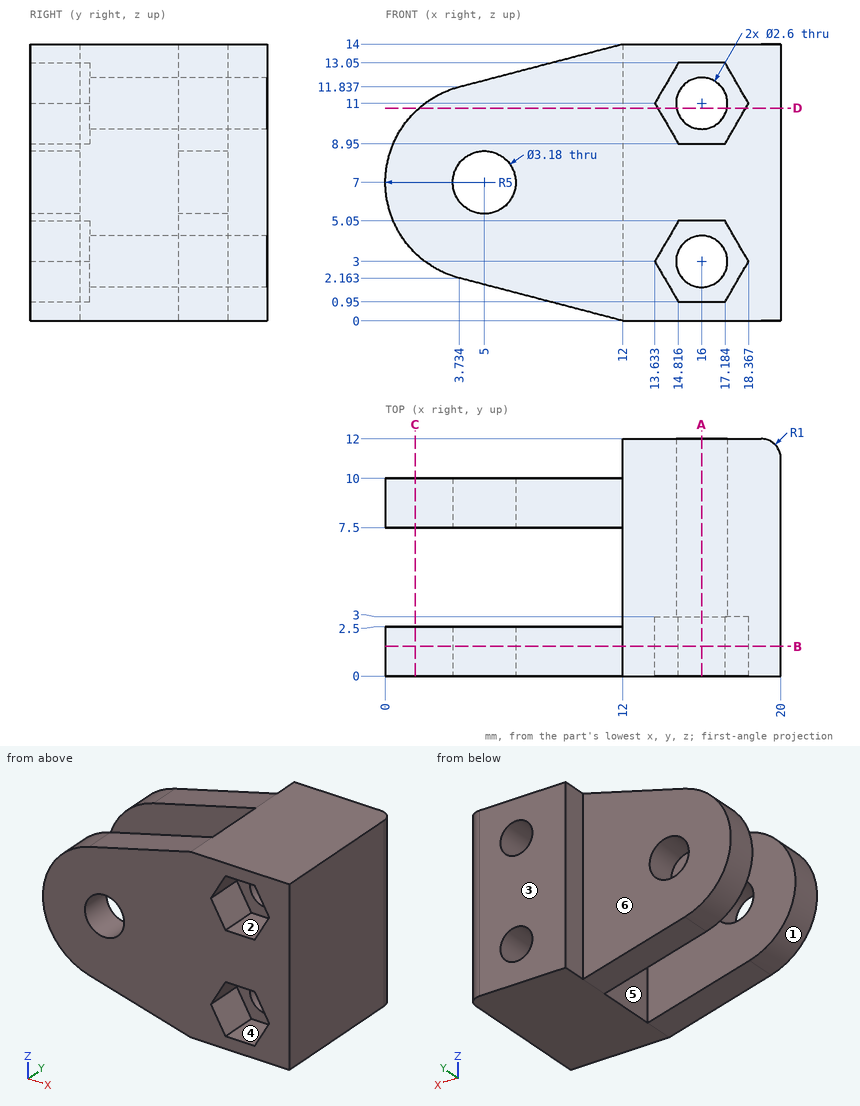
Study the drawing (mm; zero at the part's minimum x, y, z) and answer. A direction names the side the tool comes from. Give positions to 0.01 mm unless a question says otherwise; leave off trailing zeros. Order: outer loops, then holes, each group sorted by start corner. A loop starts at its lowest first (then second) coordinate and runs counter-clockwise, first axis right, second up. Notation, with made-up numbers: (-37.5, 54.25) - (-30.5, 54.25) arc R23 cw to (-30.5, 66.25) - close; hole circle Ø9 at (-29, 83). An arc over 180 degrees is marked (long way). Answer in a Markdown table with one row per item. Add a question column.
Q1. Which of the six approach directions +Z, -Z, +X, -X, +Y, -Y give full straight-line access (tool end or side, diameter ignored) to the marked faces 4, 5 and 6?
Q2. The part is cut by section B-B (y = 1.5). Give the number of separate pieces and of enclosed holes in the cut face.
Q3. The part is cut by section C-C (x = 1.5). Determine the outline of the cut face in (y, z), then the cut area to 3 significant figures.
Q4. Find the intervals of material crossed by line 1 along Z through (x, y) = (16, 9.25); line 2 along Z through (x, y) = (16.25, 1.5); line 3 along Y through (x, z) = (7.75, 6), in increasing order. Write a range as [from, to].
Q5. For a pull along X with two mould halves and no side action, classify the marked faces 1, 2 and 3 as released by +X, released by -X, zero draft, split by the parting line, or undercut.
Q6. The part is cut by section D-D (z = 10.75). Determine the outline of the cut face in (x, y) (1 decimal).
Q7. The part is cut by section A-A (x = 16). Determine the outline of the cut face in (y, z).
Q8. Given P1, Ø5, axis at x = 2, z = 8.5, coming from the +Y side; P2, Ø4, axis at x = 8, y = 7.5, coming from the -Z side; P3, Ø1, axis at y = 11, z = 6, coming from the -X side, each flat-ended and moving along its own axis, determine where each tip first touches the part or whether it passes through.
Determined:
| question | item | result |
|---|---|---|
| 1 | face 4 | -Y |
| 1 | face 5 | +Z, -Z, -X |
| 1 | face 6 | +Z, -Z, -X, +Y |
| 2 | separate pieces | 1 |
| 2 | enclosed holes | 3 |
| 3 | outline | (0, 3.43) - (2.5, 3.43) - (2.5, 10.57) - (0, 10.57) - close; (7.5, 3.43) - (10, 3.43) - (10, 10.57) - (7.5, 10.57) - close |
| 3 | area | 35.7 mm² |
| 4 | line 1 | z = [0, 1.7], [4.3, 9.7], [12.3, 14] |
| 4 | line 2 | z = [0, 0.95], [5.05, 8.95], [13.05, 14] |
| 4 | line 3 | y = [0, 2.5], [7.5, 10] |
| 5 | face 1 | released by -X |
| 5 | face 2 | undercut |
| 5 | face 3 | zero draft |
| 6 | outline | (1.7, 0) - (13.8, 0) - (13.8, 3) - (14.7, 3) - (14.7, 12) - (12, 12) - (12, 10) - (1.7, 10) - (1.7, 7.5) - (12, 7.5) - (12, 2.5) - (1.7, 2.5) - close; (17.3, 3) - (18.2, 3) - (18.2, 0) - (20, 0) - (20, 11) arc R1 ccw to (19, 12) - (17.3, 12) - close |
| 7 | outline | (0, 0) - (12, 0) - (12, 1.7) - (3, 1.7) - (3, 0.95) - (0, 0.95) - close; (0, 5.05) - (3, 5.05) - (3, 4.3) - (12, 4.3) - (12, 9.7) - (3, 9.7) - (3, 8.95) - (0, 8.95) - close; (0, 13.05) - (3, 13.05) - (3, 12.3) - (12, 12.3) - (12, 14) - (0, 14) - close |
| 8 | P1 | stops at y = 10 |
| 8 | P2 | stops at z = 0.52 |
| 8 | P3 | stops at x = 12 |
